Autodesk Inventor part; units mm, degrees
ref_plane "YZ Plane" through (0, 0, 0) normal (1, 0, 0) x (0, 1, 0)
ref_plane "XZ Plane" through (0, 0, 0) normal (0, 1, 0) x (-1, 0, 0)
ref_plane "XY Plane" through (0, 0, 0) normal (0, 0, 1) x (1, 0, 0)
sketch "Sketch1" plane through (0, 0, 0) normal (0, 0, 1) x (1, 0, 0)
  line L0 (0, 0) -> (38.1, 0)
  line L1 (38.1, 0) -> (38.1, 38.1)
  line L2 (38.1, 38.1) -> (0, 38.1)
  line L3 (0, 38.1) -> (0, 0)
  dimension "d0" = 38.1
  dimension "d1" = 38.1
extrude "Extrusion1" add sketch "Sketch1" along normal blind 38.1
sketch "Sketch2" plane through (0, 0, 38.1) normal (0, 0, 1) x (1, 0, 0)
  line L0 (6.35, 6.35) -> (32.004, 6.35)
  line L1 (32.004, 6.35) -> (32.004, 32.004)
  line L2 (32.004, 32.004) -> (6.35, 32.004)
  line L3 (6.35, 32.004) -> (6.35, 6.35)
  line L4 (38.1, 0) -> (38.1, 38.1)
  line L5 (0, 0) -> (38.1, 0)
  line L6 (38.1, 0) -> (38.1, 38.1)
  line L7 (38.1, 38.1) -> (0, 38.1)
  line L8 (0, 38.1) -> (0, 0)
  dimension "d4" = 25.654
  dimension "d5" = 25.654
extrude "Extrusion2" cut sketch "Sketch2" against normal blind 31.75 contours L3 L2 L1 L0
sketch "Sketch5" plane through (0, 0, 38.1) normal (0, 0, 1) x (1, 0, 0)
  line L0 (6.35, 6.35) -> (6.35, 32.004)
  line L1 (6.35, 6.35) -> (32.004, 6.35)
  line L2 (32.004, 6.35) -> (32.004, 32.004)
  line L3 (32.004, 32.004) -> (6.35, 32.004)
  line L4 (6.35, 32.004) -> (6.35, 6.35)
  line L5 (0, 0) -> (38.1, 0)
  line L6 (0, 0) -> (38.1, 0)
  line L7 (38.1, 0) -> (38.1, 38.1)
  line L8 (38.1, 38.1) -> (0, 38.1)
  line L9 (0, 38.1) -> (0, 0)
extrude "Extrusion4" add sketch "Sketch5" along normal blind 38.1
sketch "Sketch7" plane through (38.1, 0, 0) normal (1, 0, 0) x (0, 0, -1)
  line L0 (0, 0) -> (-76.2, 0)
  line L1 (0, 0) -> (-38.1, 0)
  line L2 (-38.1, 0) -> (-38.1, 38.1)
  line L3 (-38.1, 38.1) -> (0, 38.1)
  line L4 (0, 38.1) -> (0, 0)
  line L5 (-76.2, 6.35) -> (-6.35, 6.35)
  line L6 (-6.35, 6.35) -> (-32.004, 6.35)
  line L7 (-32.004, 6.35) -> (-32.004, 32.004)
  line L8 (-32.004, 32.004) -> (-6.35, 32.004)
  line L9 (-6.35, 32.004) -> (-6.35, 6.35)
  dimension "d16" = 38.1
  dimension "d17" = 38.1
  dimension "d20" = 25.654
  dimension "d21" = 25.654
extrude "Extrusion6" add sketch "Sketch7" along normal blind 38.1
sketch "Sketch9" plane through (38.1, 6.35, 6.35) normal (1, 0, 0) x (0, 0, -1)
  line L0 (-25.654, 0) -> (-25.654, 25.654)
  line L1 (0, 0) -> (0, 25.654)
  line L2 (-25.654, 0) -> (0, 0)
  line L3 (0, 0) -> (0, 25.654)
  line L4 (0, 25.654) -> (-25.654, 25.654)
  line L5 (-25.654, 25.654) -> (-25.654, 0)
  point P0 (6.35, -6.35)
extrude "Extrusion7" cut sketch "Sketch9" against normal blind 31.75
sketch "Sketch10" plane through (0, 38.1, 76.2) normal (0, 1, 0) x (1, 0, 0)
  line L0 (76.2, 69.85) -> (6.35, 69.85)
  line L1 (6.35, 69.85) -> (32.004, 69.85)
  line L2 (32.004, 69.85) -> (32.004, 44.196)
  line L3 (32.004, 44.196) -> (6.35, 44.196)
  line L4 (6.35, 44.196) -> (6.35, 69.85)
  line L5 (38.1, 38.1) -> (38.1, 0)
  line L6 (0, 76.2) -> (0, 0)
  line L7 (38.1, 38.1) -> (0, 38.1)
  line L8 (0, 38.1) -> (0, 76.2)
  line L9 (0, 76.2) -> (38.1, 76.2)
  line L10 (38.1, 76.2) -> (38.1, 38.1)
  point P0 (0, 38.1)
  dimension "d26" = 25.654
  dimension "d27" = 25.654
extrude "Extrusion8" add sketch "Sketch10" along normal blind 38.1
sketch "Sketch11" plane through (6.35, 38.1, 6.35) normal (0, 1, 0) x (1, 0, 0)
  line L0 (0, -25.654) -> (25.654, -25.654)
  line L1 (25.654, -25.654) -> (0, -25.654)
  line L2 (0, -25.654) -> (0, 0)
  line L3 (0, 0) -> (25.654, 0)
  line L4 (25.654, 0) -> (25.654, -25.654)
  point P0 (-6.35, 6.35)
extrude "Extrusion9" cut sketch "Sketch11" against normal blind 6.35
sketch "Sketch12" plane through (0, 76.2, 76.2) normal (0, 1, 0) x (1, 0, 0)
  line L0 (38.1, 55.88) -> (32.004, 55.88)
  line L1 (32.004, 55.88) -> (32.004, 58.42)
  line L2 (32.004, 58.42) -> (38.1, 58.42)
  line L3 (38.1, 58.42) -> (38.1, 55.88)
  point P0 (0, 76.2)
  dimension "d32" = 6.096
  dimension "d33" = 2.54
extrude "Extrusion10" cut sketch "Sketch12" against normal blind 38.1
sketch "Sketch13" plane through (76.2, 38.1, 38.1) normal (0, 1, 0) x (1, 0, 0)
  line L0 (0, 31.75) -> (0, 6.096)
  line L1 (-44.196, 17.78) -> (0, 17.78)
  line L2 (0, 17.78) -> (0, 20.32)
  line L3 (0, 20.32) -> (-44.196, 20.32)
  line L4 (-44.196, 20.32) -> (-44.196, 17.78)
  point P0 (-76.2, 38.1)
  dimension "d36" = 2.54
extrude "Extrusion11" cut sketch "Sketch13" against normal blind 6.35
sketch "Sketch15" plane through (0, 76.2, 76.2) normal (0, 1, 0) x (1, 0, 0)
  line L0 (17.78, 38.1) -> (20.32, 38.1)
  line L1 (20.32, 38.1) -> (20.32, 44.196)
  line L2 (20.32, 44.196) -> (17.78, 44.196)
  line L3 (17.78, 44.196) -> (17.78, 38.1)
  point P0 (0, 76.2)
  dimension "d39" = 2.54
  dimension "d40" = 6.096
extrude "Extrusion12" cut sketch "Sketch15" against normal blind 38.1
sketch "Sketch16" plane through (0, 38.1, 76.2) normal (0, 1, 0) x (1, 0, 0)
  line L0 (20.32, 44.196) -> (20.32, 38.1)
  line L1 (0, 0) -> (38.1, 0)
  line L2 (20.32, 44.196) -> (17.78, 44.196)
  line L3 (17.78, 44.196) -> (17.78, 0)
  line L4 (17.78, 0) -> (20.32, 0)
  line L5 (20.32, 0) -> (20.32, 44.196)
  point P0 (0, 76.2)
  dimension "d43" = 2.54
extrude "Extrusion13" cut sketch "Sketch16" against normal blind 6.35
sketch "Sketch17" plane through (38.1, 0, 76.2) normal (1, 0, 0) x (0, 0, -1)
  line L0 (38.1, 0) -> (38.1, 38.1)
  line L1 (0, 17.78) -> (38.1, 17.78)
  line L2 (38.1, 17.78) -> (38.1, 20.32)
  line L3 (38.1, 20.32) -> (0, 20.32)
  line L4 (0, 20.32) -> (0, 17.78)
  point P0 (76.2, 0)
  dimension "d46" = 2.54
extrude "Extrusion14" cut sketch "Sketch17" against normal blind 6.35
sketch "Sketch18" plane through (38.1, 0, 38.1) normal (0, 0, 1) x (1, 0, 0)
  line L0 (0, 17.78) -> (38.1, 17.78)
  line L1 (38.1, 17.78) -> (38.1, 20.32)
  line L2 (38.1, 20.32) -> (0, 20.32)
  line L3 (0, 20.32) -> (0, 17.78)
  point P0 (-38.1, 0)
  dimension "d49" = 38.1
  dimension "d50" = 2.54
extrude "Extrusion15" cut sketch "Sketch18" against normal blind 6.35
sketch "Sketch20" plane through (38.1, 38.1, 38.1) normal (0, 0, 1) x (1, 0, 0)
  line L0 (-17.78, -6.096) -> (-17.78, 38.1)
  line L1 (0, 0) -> (-17.78, 0)
  line L2 (-17.78, 38.1) -> (-16.51, 38.1)
  line L3 (-16.51, 38.1) -> (-16.51, 0)
  line L4 (-16.51, 0) -> (-17.78, 0)
  line L5 (-17.78, 0) -> (-17.78, 38.1)
  point P0 (-38.1, -38.1)
  dimension "d53" = 1.27
extrude "Extrusion16" cut sketch "Sketch20" against normal blind 6.35
sketch "Sketch21" plane through (38.1, 38.1, 76.2) normal (0, 1, 0) x (1, 0, 0)
  line L0 (-17.78, 0) -> (-17.78, 44.196)
  line L1 (0, 0) -> (-17.78, 0)
  line L2 (-17.78, 44.196) -> (-16.51, 44.196)
  line L3 (-16.51, 44.196) -> (-16.51, 0)
  line L4 (-16.51, 0) -> (-17.78, 0)
  line L5 (-17.78, 0) -> (-17.78, 44.196)
  point P0 (-38.1, 76.2)
  dimension "d56" = 1.27
extrude "Extrusion17" cut sketch "Sketch21" against normal blind 6.35
sketch "Sketch23" plane through (0, 38.1, 38.1) normal (0, 0, 1) x (1, 0, 0)
  line L0 (17.78, 0) -> (17.78, 38.1)
  line L1 (17.78, 0) -> (0, 0)
  line L2 (17.78, 38.1) -> (16.51, 38.1)
  line L3 (16.51, 38.1) -> (16.51, 0)
  line L4 (16.51, 0) -> (17.78, 0)
  line L5 (17.78, 0) -> (17.78, 38.1)
  point P0 (0, -38.1)
  dimension "d59" = 1.27
extrude "Extrusion18" cut sketch "Sketch23" against normal blind 6.35
sketch "Sketch24" plane through (0, 38.1, 76.2) normal (0, 1, 0) x (1, 0, 0)
  line L0 (17.78, 44.196) -> (17.78, 0)
  line L1 (17.78, 0) -> (0, 0)
  line L2 (17.78, 44.196) -> (16.51, 44.196)
  line L3 (16.51, 44.196) -> (16.51, 0)
  line L4 (16.51, 0) -> (17.78, 0)
  line L5 (17.78, 0) -> (17.78, 44.196)
  point P0 (0, 76.2)
  dimension "d62" = 1.27
extrude "Extrusion19" cut sketch "Sketch24" against normal blind 6.35
sketch "Sketch25" plane through (38.1, 0, 76.2) normal (1, 0, 0) x (0, 0, -1)
  line L0 (38.1, 0) -> (38.1, 17.78)
  line L1 (38.1, 17.78) -> (0, 17.78)
  line L2 (0, 17.78) -> (0, 16.51)
  line L3 (0, 16.51) -> (38.1, 16.51)
  line L4 (38.1, 16.51) -> (38.1, 17.78)
  point P0 (76.2, 0)
  dimension "d65" = 38.1
  dimension "d66" = 1.27
extrude "Extrusion20" cut sketch "Sketch25" against normal blind 6.35
sketch "Sketch26" plane through (38.1, 38.1, 76.2) normal (1, 0, 0) x (0, 0, -1)
  line L0 (0, -17.78) -> (38.1, -17.78)
  line L1 (38.1, -17.78) -> (0, -17.78)
  line L2 (0, -17.78) -> (0, -16.51)
  line L3 (0, -16.51) -> (38.1, -16.51)
  line L4 (38.1, -16.51) -> (38.1, -17.78)
  point P0 (76.2, -38.1)
  dimension "d69" = 38.1
  dimension "d70" = 1.27
extrude "Extrusion21" cut sketch "Sketch26" against normal blind 6.35
sketch "Sketch27" plane through (38.1, 0, 38.1) normal (0, 0, 1) x (1, 0, 0)
  line L0 (0, 21.59) -> (0, 38.1)
  line L1 (0, 20.32) -> (38.1, 20.32)
  line L2 (0, 21.59) -> (38.1, 21.59)
  line L3 (38.1, 21.59) -> (38.1, 20.32)
  line L4 (38.1, 20.32) -> (0, 20.32)
  line L5 (0, 20.32) -> (0, 21.59)
  line L6 (38.1, 17.78) -> (0, 17.78)
  line L7 (0, 17.78) -> (38.1, 17.78)
  line L8 (38.1, 17.78) -> (38.1, 16.51)
  line L9 (38.1, 16.51) -> (0, 16.51)
  line L10 (0, 16.51) -> (0, 17.78)
  point P0 (-38.1, 0)
  dimension "d73" = 38.1
  dimension "d74" = 1.27
extrude "Extrusion22" cut sketch "Sketch27" against normal blind 6.35
sketch "Sketch28" plane through (38.1, 38.1, 38.1) normal (0, 1, 0) x (1, 0, 0)
  line L0 (0, 20.32) -> (38.1, 20.32)
  line L1 (0, 20.32) -> (38.1, 20.32)
  line L2 (38.1, 20.32) -> (38.1, 21.59)
  line L3 (38.1, 21.59) -> (0, 21.59)
  line L4 (0, 21.59) -> (0, 20.32)
  line L5 (-6.096, 17.78) -> (38.1, 17.78)
  line L6 (38.1, 17.78) -> (0, 17.78)
  line L7 (0, 17.78) -> (0, 16.51)
  line L8 (0, 16.51) -> (38.1, 16.51)
  line L9 (38.1, 16.51) -> (38.1, 17.78)
  point P0 (-38.1, 38.1)
  point P1 (0, 17.78)
  dimension "d77" = 38.1
  dimension "d78" = 1.27
  dimension "d79" = 38.1
  dimension "d80" = 1.27
extrude "Extrusion23" cut sketch "Sketch28" against normal blind 6.35
sketch "Sketch29" plane through (38.1, 38.1, 0) normal (1, 0, 0) x (0, 0, -1)
  line L0 (-17.78, -6.096) -> (-6.35, -6.096)
  line L1 (-6.35, 38.1) -> (-17.78, 38.1)
  line L2 (-17.78, -6.096) -> (-16.51, -6.096)
  line L3 (-16.51, -6.096) -> (-16.51, 38.1)
  line L4 (-16.51, 38.1) -> (-17.78, 38.1)
  line L5 (-17.78, 38.1) -> (-17.78, -6.096)
  line L6 (-21.59, 0) -> (-21.59, -6.096)
  line L7 (-20.32, 38.1) -> (-20.32, -6.096)
  line L8 (-21.59, -6.096) -> (-20.32, -6.096)
  line L9 (-20.32, -6.096) -> (-20.32, 38.1)
  line L10 (-20.32, 38.1) -> (-21.59, 38.1)
  line L11 (-21.59, 38.1) -> (-21.59, -6.096)
  point P0 (0, -38.1)
  point P1 (-20.32, -6.096)
  dimension "d83" = 1.27
extrude "Extrusion24" cut sketch "Sketch29" against normal blind 6.35
sketch "Sketch30" plane through (76.2, 38.1, 21.59) normal (0, 0, -1) x (-1, 0, 0)
  line L0 (0, 0) -> (38.1, 0)
  line L1 (44.196, 38.1) -> (44.196, -6.096)
  line L2 (38.1, 0) -> (44.196, 0)
  line L3 (44.196, 0) -> (44.196, -6.096)
  line L4 (44.196, -6.096) -> (38.1, -6.096)
  line L5 (38.1, -6.096) -> (38.1, 0)
  point P0 (76.2, -38.1)
  point P1 (44.196, 0)
extrude "Extrusion25" add sketch "Sketch30" along normal blind 5.08
sketch "Sketch31" plane through (21.59, 38.1, 38.1) normal (-1, 0, 0) x (0, 0, 1)
  line L0 (38.1, -6.096) -> (-6.096, -6.096)
  line L1 (0, 0) -> (-6.096, 0)
  line L2 (-6.096, 0) -> (-6.096, -6.096)
  line L3 (-6.096, -6.096) -> (0, -6.096)
  line L4 (0, -6.096) -> (0, 0)
  point P0 (-38.1, -38.1)
extrude "Extrusion26" add sketch "Sketch31" along normal blind 5.08
sketch "Sketch32" plane through (0, 0, 76.2) normal (-1, 0, 0) x (0, 0, 1)
  line L0 (0, 38.1) -> (0, 0)
  line L1 (0, 19.05) -> (-76.2, 19.05)
  line L2 (-76.2, 19.05) -> (-76.2, 0)
  line L3 (-76.2, 0) -> (0, 0)
  line L4 (0, 0) -> (0, 19.05)
  line L5 (-76.2, 0) -> (-56.896, 0)
  line L6 (-56.896, 0) -> (-56.896, 76.2)
  line L7 (-56.896, 76.2) -> (-76.2, 76.2)
  line L8 (-76.2, 76.2) -> (-76.2, 0)
  point P0 (0, 0)
  point P1 (-56.896, 19.05)
  dimension "d90" = 19.304
  dimension "d91" = 76.2
extrude "Extrusion27" add sketch "Sketch32" along normal blind 12.7 contours L0 L3 L6 L1 | L6 L3 L2 L1
sketch "Sketch34" plane through (-12.7, 0, 76.2) normal (-1, 0, 0) x (0, 0, 1)
  line L0 (0, 38.1) -> (0, 19.05)
  line L1 (0, 19.05) -> (-76.2, 19.05)
  line L2 (-76.2, 19.05) -> (-76.2, 38.1)
  line L3 (-76.2, 38.1) -> (0, 38.1)
  line L4 (0, 38.1) -> (0, 19.05)
  point P0 (-76.2, 0)
  dimension "d98" = 76.2
  dimension "d99" = 19.05
extrude "Extrusion29" add sketch "Sketch34" against normal blind 6.35
sketch "Sketch35" plane through (-12.7, 0, 76.2) normal (-1, 0, 0) x (0, 0, 1)
  line L0 (-76.2, 0) -> (-95.25, 0)
  line L1 (-95.25, 0) -> (-95.25, 76.2)
  line L2 (-95.25, 76.2) -> (-76.2, 76.2)
  line L3 (-76.2, 76.2) -> (-76.2, 0)
  dimension "d102" = 19.05
  dimension "d103" = 76.2
extrude "Extrusion30" add sketch "Sketch35" against normal blind 6.35
sketch "Sketch37" plane through (0, 19.05, 76.2) normal (0, 1, 0) x (1, 0, 0)
  line L0 (0, 76.2) -> (-6.35, 76.2)
  line L1 (-6.35, 76.2) -> (-6.35, 95.25)
  line L2 (-6.35, 95.25) -> (0, 95.25)
  line L3 (0, 95.25) -> (0, 76.2)
  dimension "d106" = 6.35
  dimension "d107" = 19.05
extrude "Extrusion31" add sketch "Sketch37" against normal blind 19.05
sketch "Sketch38" plane through (38.1, 0, 38.1) normal (0, -1, 0) x (1, 0, 0)
  line L0 (-38.1, -38.1) -> (-31.75, -38.1)
  line L1 (-31.75, -38.1) -> (-31.75, -57.15)
  line L2 (-31.75, -57.15) -> (-38.1, -57.15)
  line L3 (-38.1, -57.15) -> (-38.1, -38.1)
  dimension "d110" = 6.35
  dimension "d111" = 19.05
extrude "Extrusion32" add sketch "Sketch38" against normal blind 76.2
sketch "Sketch39" plane through (-12.7, 0, 76.2) normal (-1, 0, 0) x (0, 0, 1)
  circle A0 centre (-86.36, 50.8) radius 3.81
  point P0 (-76.2, 0)
  dimension "d114" = 7.62
extrude "Extrusion33" cut sketch "Sketch39" against normal through all
properties part number "corner connector with rails (front right)"
Build history of the part. All positions in model axes, mm. A direction names the side the tool comes from. Coordinates: 2 decimals unless noted, no trailing zeros. Order: outer loops, then holes, each group sorted by start corner. A loop starts at its lowest first (then second) coordinate and runs counter-clockwise, first axis right, second up. Notation, with made-up numbers: M -17,53.5 L 1,53.5 A23 ccw 1,61.5 Z; hole C 17.5,-32 d7. An arc over 180 degrees is marked long. One line per question, with ' | ' between items. Start each with the question number.
Q1. Saw through at B-B (z = 27.5). List the corners of the cut face in (x, y).
Q2. 3-axis set-ups, long thin cutter, end or side, ignore diameter. For faces 4 (the face through (57, 35, 21.59)), 5 (the face through (6.35, 33, 26)), 6 (the face through (57, 8, 38.1)): which of +Z, -Z, +X, -X, +Y, -Y reach the whole face in a straight line?
Q3. Saw through at C-C (z = -10.16). List the corners of the cut face in (x, y), then the cut area to 3 significant figures.
Q4. Saw through at D-D (x = 42). List the corners of the cut face in (y, z).
Q5. Probe L1, parallel to X at y = 25.5, z = 42.5; L2, parallel to Y at x = -9, z = -10; L3, parallel to X at y = 38, z = 47. List the from-to ranges inside material, lowest first. Write a range as from..to.
Q6. Saw through at A-A (y = 36.5). List the corners of the cut face in (x, z), then the cut area to 3 significant figures.
Q7. Flat gauge pins, fed straight in: pin 1 Ø13 at (x, z) = (26, 61) entering from +Y; pin 2 Ø5 at (y, z) = (51, 32) entering from +X; pin 3 Ø7 at (x, y) = (-8.5, 64) entering from +Z. Where does each tip first touch, or does it go through?
Q8. Two-plate mould, pull along X, no slides. Class faces 1 (the face through (19, 38.1, 35)), 2 (the face through (38.1, 30, 57)), 3 (the face through (57, 38.1, 8)): +X half, -X half, draft (parallel to the pull), parting line (faces both ways), or undercut.
Check values:
1) outline: M -12.7,0 L 76.2,0 L 76.2,6.35 L 6.35,6.35 L 6.35,76.2 L 0,76.2 L 0,19.05 L -6.35,19.05 L -6.35,38.1 L -12.7,38.1 Z; M 32,32 L 76.2,32 L 76.2,38.1 L 38.1,38.1 L 38.1,76.2 L 32,76.2 Z
2) face 4: +X, +Y | face 5: none | face 6: +Z, +X, +Y, -Y
3) outline: M -12.7,0 L 6.35,0 L 6.35,46.99 L 0,46.99 L 0,19.05 L -6.35,19.05 L -6.35,46.99 L -12.7,46.99 Z; M -12.7,54.61 L -6.35,54.61 L -6.35,76.2 L -12.7,76.2 Z; M 0,54.61 L 6.35,54.61 L 6.35,76.2 L 0,76.2 Z | area: 992 mm2
4) outline: M 0,0 L 38.1,0 L 38.1,16.51 L 32,16.51 L 32,6.35 L 6.35,6.35 L 6.35,32 L 16.51,32 L 16.51,38.1 L 0,38.1 Z; M 21.59,32 L 32,32 L 32,21.59 L 38.1,21.59 L 38.1,38.1 L 21.59,38.1 Z
5) L1: x = -12.7..-6.35, 0..6.35, 32..38.1 | L2: y = 0..46.99, 54.61..76.2 | L3: x = -12.7..-6.35, 0..16.51, 21.59..38.1
6) outline: M -12.7,-19.05 L -6.35,-19.05 L -6.35,76.2 L -12.7,76.2 Z; M 0,-19.05 L 6.35,-19.05 L 6.35,0 L 76.2,0 L 76.2,16.51 L 38.1,16.51 L 38.1,21.59 L 76.2,21.59 L 76.2,38.1 L 38.1,38.1 L 38.1,76.2 L 21.59,76.2 L 21.59,38.1 L 16.51,38.1 L 16.51,76.2 L 0,76.2 Z; hole M 6.35,6.35 L 32,6.35 L 32,32 L 6.35,32 Z | area: 4,040 mm2
7) pin 1: stops at y = 38.1 | pin 2: stops at x = 38.1 | pin 3: stops at z = 0
8) face 1: undercut | face 2: +X half | face 3: draft
